Autodesk Inventor part; units mm, degrees
ref_plane "ANBAU_XY" through (0, 0, 40) normal (0, 0, 1) x (1, 0, 0)
ref_plane "ANBAU_YZ" through (0, 0, 40) normal (1, 0, 0) x (0, 1, 0)
ref_plane "ANBAU_ZX" through (0, 0, 40) normal (0, 1, 0) x (0, 0, 1)
sketch "Sketch_14" plane through (0, 0, 0) normal (1, 0, 0) x (0, 1, 0)
  line L0 (0, -26.1) -> (0, 0)
  line L1 (0, 0) -> (3.2, 0)
  arc A0 (3.5, -0.3) -> (3.2, 0) centre (3.2, -0.3) ccw
  line L2 (3.5, -0.3) -> (3.5, -1.5)
  arc A1 (3.5, -1.5) -> (3.5, -3.5) centre (6.3284, -2.5) ccw
  line L3 (3.5, -3.5) -> (3.5, -4.5)
  arc A2 (3.5, -4.5) -> (3.5, -5.9) centre (5.4799, -5.2) ccw
  line L4 (3.5, -5.9) -> (3.5, -6.9)
  arc A3 (3.5, -6.9) -> (3.5, -7.9) centre (4.9142, -7.4) ccw
  line L5 (3.5, -7.9) -> (3.5, -8.9)
  arc A4 (3.5, -8.9) -> (3.5, -9.5) centre (4.3485, -9.2) ccw
  line L6 (3.5, -9.5) -> (3.5, -10.5)
  line L7 (3.5, -10.5) -> (4.25, -15.9)
  line L8 (4.25, -15.9) -> (4.25, -26.1)
  line L9 (4.25, -26.1) -> (0, -26.1)
  line L10 (0, -26.1) -> (0, 0)
revolve "Revolution1" add sketch "Sketch_14" angle 360 about axis through (0, 0, -26.1) along (0, 0, -1)
sketch "Sketch_13" plane through (0, 0, -21) normal (0, 0, 1) x (1, 0, 0)
  line L0 (5, -1.85) -> (-5, -1.85)
  circle A0 centre (0, 3.9556) radius 0.6944
revolve "Revolution2" add sketch "Sketch_13" angle 80 mid plane about axis through (5, -1.85, -21) along (-1, 0, 0)
sketch "Sketch_15" plane through (0, 0, -21) normal (0, 0, 1) x (1, 0, 0)
  line L0 (-5, 1.85) -> (5, 1.85)
  circle A0 centre (0, -3.9556) radius 0.6944
revolve "Revolution3" add sketch "Sketch_15" angle 80 mid plane about axis through (-5, 1.85, -21) along (1, 0, 0)
sketch "Sketch_7" plane through (0, 0, 0) normal (1, 0, 0) x (0, 1, 0)
  line L0 (0, -41.1) -> (0, -26.1)
  line L1 (0, -26.1) -> (2.95, -26.1)
  line L2 (2.95, -26.1) -> (2.95, -28.6)
  line L3 (2.95, -28.6) -> (3.15, -28.6)
  line L4 (3.15, -28.6) -> (3.15, -39.35)
  line L5 (3.15, -39.35) -> (3.45, -39.35)
  line L6 (3.45, -39.35) -> (3.45, -41.1)
  line L7 (3.45, -41.1) -> (2.9, -41.1)
  line L8 (2.9, -41.1) -> (2.9, -40.8)
  line L9 (2.9, -40.8) -> (0, -40.8)
  line L10 (0, -40.8) -> (0, -26.1)
revolve "Revolution4" add sketch "Sketch_7" angle 360 about axis through (0, 0, -41.1) along (0, 0, -1)
sketch "Sketch_8" plane through (0, 0, 0) normal (1, 0, 0) x (0, 1, 0)
  line L0 (0, -39.35) -> (0, -27.45)
  line L1 (0, -27.45) -> (4.05, -27.45)
  line L2 (4.05, -27.45) -> (4.775, -28.175)
  line L3 (4.775, -28.175) -> (4.775, -30.45)
  line L4 (4.775, -30.45) -> (4.975, -30.45)
  line L5 (4.975, -30.45) -> (4.975, -33.25)
  line L6 (4.975, -33.25) -> (4.2, -33.25)
  arc A0 (4.2, -33.25) -> (4, -33.45) centre (4.2, -33.45) ccw
  line L7 (4, -33.45) -> (4, -39.1379)
  line L8 (4, -39.1379) -> (3.7879, -39.35)
  line L9 (3.7879, -39.35) -> (0, -39.35)
  line L10 (0, -39.35) -> (0, -27.45)
revolve "Revolution5" add sketch "Sketch_8" angle 360 about axis through (0, 0, -39.35) along (0, 0, -1)
thread "Thread1"
sketch "Sketch_10" plane through (0, 0, -27.45) normal (0, 0, 1) x (1, 0, 0)
  line L0 (-8, -8) -> (8, -8)
  line L1 (8, -8) -> (8, 8)
  line L2 (8, 8) -> (-8, 8)
  line L3 (-8, 8) -> (-8, -8)
  line L4 (-4.5, -2.5981) -> (0, -5.1962)
  line L5 (0, -5.1962) -> (4.5, -2.5981)
  line L6 (4.5, -2.5981) -> (4.5, 2.5981)
  line L7 (4.5, 2.5981) -> (0, 5.1962)
  line L8 (0, 5.1962) -> (-4.5, 2.5981)
  line L9 (-4.5, 2.5981) -> (-4.5, -2.5981)
extrude "Extrusion1" cut sketch "Sketch_10" against normal blind 3
sketch "Sketch_9" plane through (0, 0, -40.8) normal (0, 0, 1) x (1, 0, 0)
  circle A0 centre (0, 0) radius 2.9
  circle A1 centre (1.75, 0) radius 0.5
  circle A2 centre (0, -1.75) radius 0.5
  circle A3 centre (-1.75, 0) radius 0.5
extrude "Extrusion2" cut sketch "Sketch_9" along normal blind 4.7
sketch "Sketch_3" plane through (0, 0, 0) normal (1, 0, 0) x (0, 1, 0)
  line L0 (0, 0) -> (0, 40)
  line L1 (0, 40) -> (1.45, 40)
  line L2 (1.45, 40) -> (1.45, 0)
  line L3 (1.45, 0) -> (0, 0)
  line L4 (0, 0) -> (0, 40)
revolve "Revolution6" add sketch "Sketch_3" angle 360 about axis through (0, 0, 0) along (0, 0, -1)
sketch "Sketch_4" plane through (0, 0, 0) normal (1, 0, 0) x (0, 1, 0)
  line L0 (1.45, 40) -> (-1.45, 40)
  line L1 (-1.45, 40) -> (-1.45, 37.1)
  line L2 (-1.45, 37.1) -> (1.45, 40)
extrude "Extrusion3" cut sketch "Sketch_4" along normal mid plane 12
ref_plane "ANBAU_XY" through (0, 0, 40) normal (0, 0, 1) x (1, 0, 0)
ref_plane "ANBAU_YZ" through (0, 0, 40) normal (1, 0, 0) x (0, 1, 0)
ref_plane "ANBAU_ZX" through (0, 0, 40) normal (0, 1, 0) x (0, 0, 1)
ref_plane "ASCF1_XY" through (0, 0, 7) normal (0, 0, 1) x (1, 0, 0)
ref_plane "ASCF1_YZ" through (0, 0, 7) normal (1, 0, 0) x (0, 1, 0)
ref_plane "ASCF1_ZX" through (0, 0, 7) normal (0, 1, 0) x (0, 0, 1)
ref_plane "CONN_XY" through (0, 0, 0) normal (0, 0, -1) x (1, 0, 0)
ref_plane "CONN_YZ" through (0, 0, 0) normal (1, 0, 0) x (0, -1, 0)
ref_plane "CONN_ZX" through (0, 0, 0) normal (0, -1, 0) x (0, 0, -1)
ref_plane "FDT_CONCAB_XY" through (0, 0, -36.1) normal (0, 0, -1) x (0, -1, 0)
ref_plane "FDT_CONCAB_YZ" through (0, 0, -36.1) normal (0, -1, 0) x (-1, 0, 0)
ref_plane "FDT_CONCAB_ZX" through (0, 0, -36.1) normal (-1, 0, 0) x (0, 0, -1)
properties part number "8082090 SDBT-M8---(stecker)"
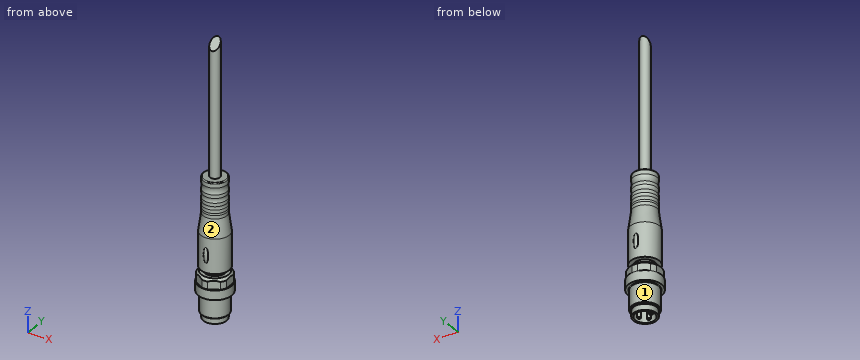
Geometry: final body of the model. Coordinates: model frame, mm. Face numbers are marked on the shaded views. A direction names the side the tool comes from. Round coordinates to 2 decimals unless told otherwise and drop trailing zeros. Order: outer loops, then holes, each group sorted by start corner. A loop starts at its lowest first (then second) coordinate and runs counter-clockwise, first axis right, second up. Notation, with made-up numbers: (-26.5, 53) -> (18.5, 53) arc R20 ccw to (18.5, 82) -> close; hole circle Ø5 at (23.25, 88). An arc over 180 degrees is marked (long way). Put each result on its own line as item: value. Start each with the question number.
Q1. Section B-B on z = 20.5. Return the cut outline in (x, y).
Q2. Line query: probe 1 along Z at (x, y) = (2.5, 2); probe 2 along Z at (x, y) = (3.5, -3.5); probe 3 along X at (y, z) = (1.25, -34). Output: solid intervals per line, ascending.
Q3. Section A-A on z = -17. Return the cut outline in (x, y).
Q4. First-contact query: pin 1 (4 mm diameter, centred on y = 3, z = -1.5, fed in from -X); pin 2 (3 mm diameter, centred on y = 0, z = -28.5, fed in from +X); pin 3 (1.1 mm diameter, centred on x = -1.5, y = 0, fed in from -Z). Flat tips, straight axial feed; report the tip coordinate or a pass-through.
Q5. Reachability of the marked faces 1 and 2 from +Z, -Z, +X, -X, +Y, -Y: full face, straight path, thin tool, end or side. Return the list, or none.
Ans:
1. outline: circle Ø2.9 at (0, 0)
2. probe 1: z = -41.1 to -27.45, -26.1 to 0
2. probe 2: z = -33.25 to -30.45
2. probe 3: x = -3.8 to 3.8
3. outline: circle Ø8.5 at (0, 0)
4. pin 1: stops at x = -3.35
4. pin 2: stops at x = 4.5
4. pin 3: stops at z = -40.8
5. face 1: -Z
5. face 2: +Z
